Part model, mm, in its own coordinate system. A direction names the side the tool comes from. Coordinates: 2 decimals unless noted, no trailing zeros. Write each loop counter-clockwise with the first axis right and the second up, starting at its lowest first coordinate (ties: lowest second). Pieces come first, ordered by that corner, then holes. Notation, with made-up numbers: (49.25, 11.5) -> (91.25, 11.5) arc R13 cw to (91.25, 19.5) -> close; hole circle Ø2 at (26, 74.5). An arc over 180 degrees is marked (long way). One line per question, with ' | ' between items. Start each with the question number.
Item 1: 3-axis set-ups, long thin cutter, end or side, ignore diameter. For faces 5 (the cylindrical face through (-2.14, 5.795, 5.07)), 6 (the flat face through (-27, 17.939, 37)), 7 (the cylindrical face through (0.1, 20.3, 4.9)), 8 (the flat face through (-53, 7, 10)): which of +Z, -Z, +X, -X, +Y, -Y reach the whole face in a straight line?
Item 2: Saw through at A-A (z = 25.5). List the corners of the cut face in (x, y), and give its area (3 significant figures).
Item 3: Pin check, flat tips, straight feed: pin 1 (5 mm diameter, centred on x = -15, y = 2.5, fed in from -Z); pin 2 (11 mm diameter, centred on x = -33, z = 39, fed in from +Y); pin 3 (6 mm diameter, centred on x = -16.5, y = 2.55, fed in from +Z); pin 4 (9 mm diameter, centred on x = -41.5, z = 17, fed in from +Y). Stop position of each tip, or through.
Item 4: Two-plate mould, pull along Z, no slides. Class faces 1 (the cylindrical face through (-54.519, -21.389, 17.508)), 2 (the flat face through (-27, -9, 43)), 3 (the cylindrical face through (-50.419, 6.403, 5.07)), 4 (the flat face through (-27, 5, 31)): pulls with the +Z half, pulls with the -Z half, needs draft (parallel to the pull), parting line crosses it, or undercut.
Item 5: Saw through at C-C (y = -20). List the corners of the cut face in (x, z).
Item 6: Saw through at B-B (x = -16.5). List the corners of the cut face in (y, z), and give its area (3 significant figures).
Item 7: Probe probe 1 along X at (y, z) = (-14, 25.5); probe 2 along Z at (x, y) = (-52, -10); probe 3 along X at (y, z) = (-18, 28). List the from-to ranges inside material, lowest first. Write a range as [from, to].
Item 8: Saw through at D-D (x = -51). List the corners of the cut face in (y, z).
from build123d import *

# Parameters (mm, degrees)
BOSS_EXTRUDE1_DEPTH            = 10
SKETCH2_W                      = 12
SKETCH2_H                      = 12.25
BOSS_EXTRUDE2_DEPTH            = 21
SKETCH4_W                      = 65
SKETCH4_H                      = 38.636969104
BOSS_EXTRUDE3_DEPTH            = 12
F_3_6_3_6_DIAMETER_HOLE1_D     = 3.6
F_3_6_3_6_DIAMETER_HOLE1_DEPTH = 10
F_3_6_3_6_DIAMETER_HOLE1_TIP   = 1.081549114
SKETCH21_W                     = 41
SKETCH21_H                     = 12.25
BOSS_EXTRUDE4_DEPTH            = 31
SKETCH23_W                     = 65
SKETCH23_H                     = 43
BOSS_EXTRUDE6_DEPTH            = 14
FILLET1_R                      = 1
F_6_6_6_6_DIAMETER_HOLE1_D     = 6.6
SKETCH28_R                     = 1.8
CUT_EXTRUDE1_DEPTH             = 44


with BuildPart() as part:
    # Sketch1 → Boss-Extrude1 (new body)
    with BuildSketch(Plane.XY):
        with BuildLine():
            Line((-6, 14.302325581), (-6, -20.697674419))
            Line((-6, -20.697674419), (6, -20.697674419))
            Line((6, -20.697674419), (6, 14.302325581))
            ThreePointArc((6, 14.302325581), (0, 20.302325581), (-6, 14.302325581))
        make_face()
    boss_extrude1 = extrude(amount=BOSS_EXTRUDE1_DEPTH)

    # Sketch2 → Boss-Extrude2 (add)
    with BuildSketch(Plane.XY.offset(10)):
        with Locations((0, -14.572674419)):
            Rectangle(SKETCH2_W, SKETCH2_H)
    boss_extrude2 = extrude(amount=BOSS_EXTRUDE2_DEPTH)

    # Sketch4 → Boss-Extrude3 (add)
    with BuildSketch(Plane.XY.offset(31)):
        with Locations((-26.5, -1.379189867)):
            Rectangle(SKETCH4_W, SKETCH4_H)
    extrude(amount=BOSS_EXTRUDE3_DEPTH)

    # Mirror2: Boss-Extrude2 across plane
    add(boss_extrude2.mirror(Plane.ZY.offset(26.5)))

    # Mirror3: Boss-Extrude1 across plane
    add(boss_extrude1.mirror(Plane.ZY.offset(26.5)))

    # Ø3.6 (3.6) Diameter Hole1
    with Locations(Plane(origin=(0, 0, 0), x_dir=(-1, 0, 0), z_dir=(0, 0, -1))):
        with Locations((1.75, 7.55218084), (1.75, -2.44781916), (51.25, 8), (51.25, -2)):
            Hole(F_3_6_3_6_DIAMETER_HOLE1_D / 2, depth=F_3_6_3_6_DIAMETER_HOLE1_DEPTH)
            with Locations((0, 0, -(F_3_6_3_6_DIAMETER_HOLE1_DEPTH + F_3_6_3_6_DIAMETER_HOLE1_TIP / 2))):  # 118° drill point
                Cone(0, F_3_6_3_6_DIAMETER_HOLE1_D / 2, F_3_6_3_6_DIAMETER_HOLE1_TIP, mode=Mode.SUBTRACT)

    # Sketch21 → Boss-Extrude4 (add)
    with BuildSketch(Plane(origin=(0, 0, 31), x_dir=(-1, 0, 0), z_dir=(0, 0, -1))):
        with Locations((26.5, -14.572674419)):
            Rectangle(SKETCH21_W, SKETCH21_H)
    extrude(amount=BOSS_EXTRUDE4_DEPTH)

    # Sketch23 → Boss-Extrude6 (add)
    with BuildSketch(Plane.XZ.offset(20.697674419)):
        with Locations((-26.5, 21.5)):
            Rectangle(SKETCH23_W, SKETCH23_H)
    extrude(amount=BOSS_EXTRUDE6_DEPTH)

    # Fillet1
    fillet1_edges = [part.edges().sort_by_distance(p)[0] for p in [
        (-26.5, -8.447674419, 31),
        (0, -8.447674419, 10),
        (-26.5, 17.939294685, 31),
        (6, 17.939294685, 37),
        (-59, 17.939294685, 37),
        (-26.5, 17.939294685, 43),
        (-53, -8.447674419, 10),
        (-6, -8.447674419, 5),
        (-47, -8.447674419, 5),
    ]]
    fillet(fillet1_edges, radius=FILLET1_R)

    # Ø6.6 (6.6) Diameter Hole1 (through all)
    with Locations(Plane(origin=(0, -34.697674419, 0), x_dir=(-1, 0, 0), z_dir=(0, -1, 0))):
        with Locations((1.1, -15.5), (1.1, -25.5), (51.9, -15.5), (51.9, -25.5)):
            Hole(F_6_6_6_6_DIAMETER_HOLE1_D / 2)

    # Sketch28 → Cut-Extrude1 (cut, through all)
    with BuildSketch(Plane.XY.offset(43)):
        with Locations((-16.5, 2.553012267)):
            Circle(SKETCH28_R)
    extrude(amount=-CUT_EXTRUDE1_DEPTH, mode=Mode.SUBTRACT)


solid = part.part
From the geometry:
1) face 5: -Z | face 6: +Z, +X, -X, +Y | face 7: -Z, +Y | face 8: +X, -X, +Y
2) outline: (-59, -34.7) -> (-55.2, -34.7) -> (-55.2, -8.45) -> (-59, -8.45) -> close; (-48.6, -34.7) -> (-4.4, -34.7) -> (-4.4, -8.45) -> (-48.6, -8.45) -> close; (2.2, -34.7) -> (6, -34.7) -> (6, -8.45) -> (2.2, -8.45) -> close | area: 1,360 mm2
3) pin 1: z = 31 | pin 2: y = 17.94 | pin 3: z = 43 | pin 4: y = -8.45
4) face 1: undercut | face 2: pulls with the +Z half | face 3: needs draft | face 4: undercut
5) outline: (-59, 0) -> (6, 0) -> (6, 43) -> (-59, 43) -> close; hole circle Ø6.6 at (-51.9, 15.5); hole circle Ø6.6 at (-51.9, 25.5); hole circle Ø6.6 at (-1.1, 15.5); hole circle Ø6.6 at (-1.1, 25.5)
6) outline: (-34.7, 0) -> (-8.45, 0) -> (-8.45, 30) arc R1 cw to (-7.45, 31) -> (0.75, 31) -> (0.75, 43) -> (-34.7, 43) -> close; (4.35, 31) -> (16.94, 31) arc R1 ccw to (17.94, 32) -> (17.94, 42) arc R1 ccw to (16.94, 43) -> (4.35, 43) -> close | area: 1,400 mm2
7) probe 1: [-59, -55.2], [-48.6, -4.4], [2.2, 6] | probe 2: [0, 12.2], [18.8, 22.2], [28.8, 43] | probe 3: [-59, -54.05], [-49.75, -3.25], [1.05, 6]
8) outline: (-34.7, 0) -> (-3.78, 0) -> (-3.78, 10) -> (-7.45, 10) arc R1 cw to (-8.45, 11) -> (-8.45, 12.33) -> (-34.7, 12.33) -> close; (-34.7, 18.67) -> (-8.45, 18.67) -> (-8.45, 22.33) -> (-34.7, 22.33) -> close; (-34.7, 28.67) -> (-8.45, 28.67) -> (-8.45, 30) arc R1 cw to (-7.45, 31) -> (16.94, 31) arc R1 ccw to (17.94, 32) -> (17.94, 42) arc R1 ccw to (16.94, 43) -> (-34.7, 43) -> close; (-0.22, 0) -> (6.22, 0) -> (6.22, 10) -> (-0.22, 10) -> close; (9.78, 0) -> (19.96, 0) -> (19.96, 10) -> (9.78, 10) -> close
